Geometry: final body of the model. Coordinates: model frame, mm. Give positions to 0.01 mm unless a question says otherwise; leave off trailing zeros. Order: outer loops, then holes, each group sorted by start corner. A loop starts at its lowest first (then second) coordinate and runs counter-clockwise, first axis right, second up. Notation, with made-up numbers: (68.25, 62.5) - (73.25, 62.5) arc R21 ccw to (73.25, 74.5) - close; hole circle Ø10 at (87, -19). An arc over 180 degrees is marked (long way). Put each result on its own line as item: value. Start each with the question number.
1. Section C-C on z = 19.25. Return the cut outline in (x, y).
2. Section D-D on x = 12. Return the cut outline in (y, z).
3. Ray query, line 1 along Z through (x, y) = (-27, 0.4); line 2 along Z through (x, y) = (-11, 3.3); line 3 along X through (y, z) = (2.4, 6.75). Return the intervals inside material, ascending. Write a range as from..to.
4. Section A-A on z = -13.75. Return the cut outline in (x, y).
5. Section B-B on x = -21.5. Return the cut outline in (y, z).
6. First-contact query: P1, Ø4.5, axis at x = -21.5, z = 19.25, coming from the -Y side; P2, Ø6, axis at x = -21.5, z = 18, coming from the +Y side. Flat tips, straight axial feed; report the tip coordinate or a pass-through.
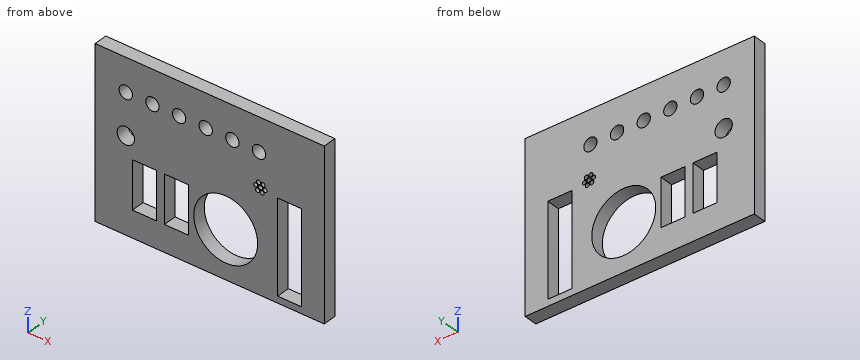
from build123d import *

# Parameters (mm, degrees)
SKICA2_W                 = 86
SKICA2_H                 = 63.5
P_IDAT_VYSUNUT_M1_DEPTH  = 5
ODEBRAT_VYSUNUT_M1_REACH = 55.685
SKICA4_R                 = 2.5
SKICA4_R_2               = 3.25
SKICA4_R_3               = 12
SKICA4_R_4               = 0.75
SKICA4_W                 = 9
SKICA4_H                 = 18
SKICA4_H_2               = 35


with BuildPart() as part:
    # Skica2 → Přidat vysunutím1 (new body)
    with BuildSketch(Plane(origin=(0, 0, 0), x_dir=(1, 0, 0), z_dir=(0, 1, 0))):
        Rectangle(SKICA2_W, SKICA2_H)
    extrude(amount=P_IDAT_VYSUNUT_M1_DEPTH)

    # Skica4 → Odebrat vysunutím1 (cut, up to next)
    with BuildSketch(Plane(origin=(0, 5, 0), x_dir=(1, 0, 0), z_dir=(0, 1, 0)), mode=Mode.PRIVATE) as odebrat_vysunut_m1_sk1:
        with Locations(Location((-31.5, -19.25, 0), (0, 0, 270))):
            Circle(SKICA4_R)
    odebrat_vysunut_m1_tool1 = extrude(odebrat_vysunut_m1_sk1.sketch, amount=-ODEBRAT_VYSUNUT_M1_REACH, mode=Mode.PRIVATE) & part.part
    # Skica4 → Odebrat vysunutím1 (cut, up to next)
    with BuildSketch(Plane(origin=(0, 5, 0), x_dir=(1, 0, 0), z_dir=(0, 1, 0)), mode=Mode.PRIVATE) as odebrat_vysunut_m1_sk2:
        with Locations(Location((-21.5, -19.25, 0), (0, 0, 270))):
            Circle(SKICA4_R)
    odebrat_vysunut_m1_tool2 = extrude(odebrat_vysunut_m1_sk2.sketch, amount=-ODEBRAT_VYSUNUT_M1_REACH, mode=Mode.PRIVATE) & part.part
    # Skica4 → Odebrat vysunutím1 (cut, up to next)
    with BuildSketch(Plane(origin=(0, 5, 0), x_dir=(1, 0, 0), z_dir=(0, 1, 0)), mode=Mode.PRIVATE) as odebrat_vysunut_m1_sk3:
        with Locations(Location((-11.5, -19.25, 0), (0, 0, 270))):
            Circle(SKICA4_R)
    odebrat_vysunut_m1_tool3 = extrude(odebrat_vysunut_m1_sk3.sketch, amount=-ODEBRAT_VYSUNUT_M1_REACH, mode=Mode.PRIVATE) & part.part
    # Skica4 → Odebrat vysunutím1 (cut, up to next)
    with BuildSketch(Plane(origin=(0, 5, 0), x_dir=(1, 0, 0), z_dir=(0, 1, 0)), mode=Mode.PRIVATE) as odebrat_vysunut_m1_sk4:
        with Locations(Location((-1.5, -19.25, 0), (0, 0, 270))):
            Circle(SKICA4_R)
    odebrat_vysunut_m1_tool4 = extrude(odebrat_vysunut_m1_sk4.sketch, amount=-ODEBRAT_VYSUNUT_M1_REACH, mode=Mode.PRIVATE) & part.part
    # Skica4 → Odebrat vysunutím1 (cut, up to next)
    with BuildSketch(Plane(origin=(0, 5, 0), x_dir=(1, 0, 0), z_dir=(0, 1, 0)), mode=Mode.PRIVATE) as odebrat_vysunut_m1_sk5:
        with Locations(Location((8.5, -19.25, 0), (0, 0, 270))):
            Circle(SKICA4_R)
    odebrat_vysunut_m1_tool5 = extrude(odebrat_vysunut_m1_sk5.sketch, amount=-ODEBRAT_VYSUNUT_M1_REACH, mode=Mode.PRIVATE) & part.part
    # Skica4 → Odebrat vysunutím1 (cut, up to next)
    with BuildSketch(Plane(origin=(0, 5, 0), x_dir=(1, 0, 0), z_dir=(0, 1, 0)), mode=Mode.PRIVATE) as odebrat_vysunut_m1_sk6:
        with Locations(Location((18.5, -19.25, 0), (0, 0, 270))):
            Circle(SKICA4_R)
    odebrat_vysunut_m1_tool6 = extrude(odebrat_vysunut_m1_sk6.sketch, amount=-ODEBRAT_VYSUNUT_M1_REACH, mode=Mode.PRIVATE) & part.part
    # Skica4 → Odebrat vysunutím1 (cut, up to next)
    with BuildSketch(Plane(origin=(0, 5, 0), x_dir=(1, 0, 0), z_dir=(0, 1, 0)), mode=Mode.PRIVATE) as odebrat_vysunut_m1_sk7:
        with Locations(Location((-31.5, -3.75, 0), (0, 0, 270))):
            Circle(SKICA4_R_2)
    odebrat_vysunut_m1_tool7 = extrude(odebrat_vysunut_m1_sk7.sketch, amount=-ODEBRAT_VYSUNUT_M1_REACH, mode=Mode.PRIVATE) & part.part
    # Skica4 → Odebrat vysunutím1 (cut, up to next)
    with BuildSketch(Plane(origin=(0, 5, 0), x_dir=(1, 0, 0), z_dir=(0, 1, 0)), mode=Mode.PRIVATE) as odebrat_vysunut_m1_sk8:
        with Locations(Location((6, 13.75, 0), (0, 0, 270))):
            Circle(SKICA4_R_3)
    odebrat_vysunut_m1_tool8 = extrude(odebrat_vysunut_m1_sk8.sketch, amount=-ODEBRAT_VYSUNUT_M1_REACH, mode=Mode.PRIVATE) & part.part
    # Skica4 → Odebrat vysunutím1 (cut, up to next)
    with BuildSketch(Plane(origin=(0, 5, 0), x_dir=(1, 0, 0), z_dir=(0, 1, 0)), mode=Mode.PRIVATE) as odebrat_vysunut_m1_sk9:
        with Locations(Location((17.948758431, -5.350932037, 0), (0, 0, 270))):
            Circle(SKICA4_R_4)
    odebrat_vysunut_m1_tool9 = extrude(odebrat_vysunut_m1_sk9.sketch, amount=-ODEBRAT_VYSUNUT_M1_REACH, mode=Mode.PRIVATE) & part.part
    # Skica4 → Odebrat vysunutím1 (cut, up to next)
    with BuildSketch(Plane(origin=(0, 5, 0), x_dir=(1, 0, 0), z_dir=(0, 1, 0)), mode=Mode.PRIVATE) as odebrat_vysunut_m1_sk10:
        with Locations(Location((19, -6.75, 0), (0, 0, 270))):
            Circle(SKICA4_R_4)
    odebrat_vysunut_m1_tool10 = extrude(odebrat_vysunut_m1_sk10.sketch, amount=-ODEBRAT_VYSUNUT_M1_REACH, mode=Mode.PRIVATE) & part.part
    # Skica4 → Odebrat vysunutím1 (cut, up to next)
    with BuildSketch(Plane(origin=(0, 5, 0), x_dir=(1, 0, 0), z_dir=(0, 1, 0)), mode=Mode.PRIVATE) as odebrat_vysunut_m1_sk11:
        with Locations(Location((19.686007584, -5.140064137, 0), (0, 0, 270))):
            Circle(SKICA4_R_4)
    odebrat_vysunut_m1_tool11 = extrude(odebrat_vysunut_m1_sk11.sketch, amount=-ODEBRAT_VYSUNUT_M1_REACH, mode=Mode.PRIVATE) & part.part
    # Skica4 → Odebrat vysunutím1 (cut, up to next)
    with BuildSketch(Plane(origin=(0, 5, 0), x_dir=(1, 0, 0), z_dir=(0, 1, 0)), mode=Mode.PRIVATE) as odebrat_vysunut_m1_sk12:
        with Locations(Location((20.737249118, -6.539132085, 0), (0, 0, 270))):
            Circle(SKICA4_R_4)
    odebrat_vysunut_m1_tool12 = extrude(odebrat_vysunut_m1_sk12.sketch, amount=-ODEBRAT_VYSUNUT_M1_REACH, mode=Mode.PRIVATE) & part.part
    # Skica4 → Odebrat vysunutím1 (cut, up to next)
    with BuildSketch(Plane(origin=(0, 5, 0), x_dir=(1, 0, 0), z_dir=(0, 1, 0)), mode=Mode.PRIVATE) as odebrat_vysunut_m1_sk13:
        with Locations(Location((20.051241501, -8.149067934, 0), (0, 0, 270))):
            Circle(SKICA4_R_4)
    odebrat_vysunut_m1_tool13 = extrude(odebrat_vysunut_m1_sk13.sketch, amount=-ODEBRAT_VYSUNUT_M1_REACH, mode=Mode.PRIVATE) & part.part
    # Skica4 → Odebrat vysunutím1 (cut, up to next)
    with BuildSketch(Plane(origin=(0, 5, 0), x_dir=(1, 0, 0), z_dir=(0, 1, 0)), mode=Mode.PRIVATE) as odebrat_vysunut_m1_sk14:
        with Locations(Location((18.313992349, -8.359935834, 0), (0, 0, 270))):
            Circle(SKICA4_R_4)
    odebrat_vysunut_m1_tool14 = extrude(odebrat_vysunut_m1_sk14.sketch, amount=-ODEBRAT_VYSUNUT_M1_REACH, mode=Mode.PRIVATE) & part.part
    # Skica4 → Odebrat vysunutím1 (cut, up to next)
    with BuildSketch(Plane(origin=(0, 5, 0), x_dir=(1, 0, 0), z_dir=(0, 1, 0)), mode=Mode.PRIVATE) as odebrat_vysunut_m1_sk15:
        with Locations(Location((17.262750814, -6.960867886, 0), (0, 0, 270))):
            Circle(SKICA4_R_4)
    odebrat_vysunut_m1_tool15 = extrude(odebrat_vysunut_m1_sk15.sketch, amount=-ODEBRAT_VYSUNUT_M1_REACH, mode=Mode.PRIVATE) & part.part
    # Skica4 → Odebrat vysunutím1 (cut, up to next)
    with BuildSketch(Plane(origin=(0, 5, 0), x_dir=(1, 0, 0), z_dir=(0, 1, 0)), mode=Mode.PRIVATE) as odebrat_vysunut_m1_sk16:
        with Locations((-24.5, 12.75)):
            Rectangle(SKICA4_W, SKICA4_H)
    odebrat_vysunut_m1_tool16 = extrude(odebrat_vysunut_m1_sk16.sketch, amount=-ODEBRAT_VYSUNUT_M1_REACH, mode=Mode.PRIVATE) & part.part
    # Skica4 → Odebrat vysunutím1 (cut, up to next)
    with BuildSketch(Plane(origin=(0, 5, 0), x_dir=(1, 0, 0), z_dir=(0, 1, 0)), mode=Mode.PRIVATE) as odebrat_vysunut_m1_sk17:
        with Locations((-12.5, 12.75)):
            Rectangle(SKICA4_W, SKICA4_H)
    odebrat_vysunut_m1_tool17 = extrude(odebrat_vysunut_m1_sk17.sketch, amount=-ODEBRAT_VYSUNUT_M1_REACH, mode=Mode.PRIVATE) & part.part
    # Skica4 → Odebrat vysunutím1 (cut, up to next)
    with BuildSketch(Plane(origin=(0, 5, 0), x_dir=(1, 0, 0), z_dir=(0, 1, 0)), mode=Mode.PRIVATE) as odebrat_vysunut_m1_sk18:
        with Locations((30, 11.75)):
            Rectangle(SKICA4_W, SKICA4_H_2)
    odebrat_vysunut_m1_tool18 = extrude(odebrat_vysunut_m1_sk18.sketch, amount=-ODEBRAT_VYSUNUT_M1_REACH, mode=Mode.PRIVATE) & part.part
    add(odebrat_vysunut_m1_tool1.solids().sort_by_distance((-31.5, 5, 19.25))[0], mode=Mode.SUBTRACT)
    add(odebrat_vysunut_m1_tool2.solids().sort_by_distance((-21.5, 5, 19.25))[0], mode=Mode.SUBTRACT)
    add(odebrat_vysunut_m1_tool3.solids().sort_by_distance((-11.5, 5, 19.25))[0], mode=Mode.SUBTRACT)
    add(odebrat_vysunut_m1_tool4.solids().sort_by_distance((-1.5, 5, 19.25))[0], mode=Mode.SUBTRACT)
    add(odebrat_vysunut_m1_tool5.solids().sort_by_distance((8.5, 5, 19.25))[0], mode=Mode.SUBTRACT)
    add(odebrat_vysunut_m1_tool6.solids().sort_by_distance((18.5, 5, 19.25))[0], mode=Mode.SUBTRACT)
    add(odebrat_vysunut_m1_tool7.solids().sort_by_distance((-31.5, 5, 3.75))[0], mode=Mode.SUBTRACT)
    add(odebrat_vysunut_m1_tool8.solids().sort_by_distance((6, 5, -13.75))[0], mode=Mode.SUBTRACT)
    add(odebrat_vysunut_m1_tool9.solids().sort_by_distance((17.948758, 5, 5.350932))[0], mode=Mode.SUBTRACT)
    add(odebrat_vysunut_m1_tool10.solids().sort_by_distance((19, 5, 6.75))[0], mode=Mode.SUBTRACT)
    add(odebrat_vysunut_m1_tool11.solids().sort_by_distance((19.686008, 5, 5.140064))[0], mode=Mode.SUBTRACT)
    add(odebrat_vysunut_m1_tool12.solids().sort_by_distance((20.737249, 5, 6.539132))[0], mode=Mode.SUBTRACT)
    add(odebrat_vysunut_m1_tool13.solids().sort_by_distance((20.051242, 5, 8.149068))[0], mode=Mode.SUBTRACT)
    add(odebrat_vysunut_m1_tool14.solids().sort_by_distance((18.313992, 5, 8.359936))[0], mode=Mode.SUBTRACT)
    add(odebrat_vysunut_m1_tool15.solids().sort_by_distance((17.262751, 5, 6.960868))[0], mode=Mode.SUBTRACT)
    add(odebrat_vysunut_m1_tool16.solids().sort_by_distance((-24.5, 5, -12.75))[0], mode=Mode.SUBTRACT)
    add(odebrat_vysunut_m1_tool17.solids().sort_by_distance((-12.5, 5, -12.75))[0], mode=Mode.SUBTRACT)
    add(odebrat_vysunut_m1_tool18.solids().sort_by_distance((30, 5, -11.75))[0], mode=Mode.SUBTRACT)


solid = part.part
Resolved:
1. outline: (-43, 0) - (-34, 0) - (-34, 5) - (-43, 5) - close; (-29, 0) - (-24, 0) - (-24, 5) - (-29, 5) - close; (-19, 0) - (-14, 0) - (-14, 5) - (-19, 5) - close; (-9, 0) - (-4, 0) - (-4, 5) - (-9, 5) - close; (1, 0) - (6, 0) - (6, 5) - (1, 5) - close; (11, 0) - (16, 0) - (16, 5) - (11, 5) - close; (21, 0) - (43, 0) - (43, 5) - (21, 5) - close
2. outline: (0, -31.75) - (5, -31.75) - (5, -24.14) - (0, -24.14) - close; (0, -3.36) - (5, -3.36) - (5, 31.75) - (0, 31.75) - close
3. line 1: -31.75..-21.75, -3.75..31.75
3. line 2: -31.75..-21.75, -3.75..16.8, 21.7..31.75
3. line 3: -43..-32.75, -30.25..16.54, 17.98..18.25, 19.75..20.02, 21.46..43
4. outline: (-43, 0) - (-29, 0) - (-29, 5) - (-43, 5) - close; (-20, 0) - (-17, 0) - (-17, 5) - (-20, 5) - close; (-8, 0) - (-6, 0) - (-6, 5) - (-8, 5) - close; (18, 0) - (25.5, 0) - (25.5, 5) - (18, 5) - close; (34.5, 0) - (43, 0) - (43, 5) - (34.5, 5) - close
5. outline: (0, -31.75) - (5, -31.75) - (5, -21.75) - (0, -21.75) - close; (0, -3.75) - (5, -3.75) - (5, 16.75) - (0, 16.75) - close; (0, 21.75) - (5, 21.75) - (5, 31.75) - (0, 31.75) - close
6. P1: through
6. P2: y = 5
